Read the model definition and answer for the solid it produces. Units are mm, in the model's axes. A direction names the side the tool comes from. Give positions to 0.01 mm unless a question says otherwise; leave off trailing zeros. Write each loop counter-clockwise with the first axis right and the second up, starting at its lowest first coordinate (ties: lowest second). Pieces come first, ordered by that corner, then holes. Notation, with made-up numbers: (-25.5, 14.25) -> (23.5, 14.25) arc R21 ccw to (23.5, 28.25) -> close; hole circle Ø8 at (-33, -21.5). An arc over 180 degrees is marked (long way). Answer as CSV lines item,"result". Start each with the question number.
1. A tool of negligible diameter and unlimited length cuts with its end or side. For faces 1 (the flat face through (-2, 128, 184)), 2 (the flat face through (-150, -2, 180)), 3 (the flat face through (-153, -2, 184)), 4 (the flat face through (-3, 2, 8)), 5 (the flat face through (-171.5, 31.5, 120.2)), from which of +Z, -Z, +X, -X, +Y, -Y can it reach the whole face along a straight path? Write none if from no direction.
2. The part is cut by section D-D, the plane y = -119. Determine the outline of the cut face in (x, z).
3. Find the intervals of material crossed by line 1 (Y direction, x = 185.25, z = 145); line 2 (Y direction, x = -20, z = 146.5); line 3 (X direction, y = 103.5, z = 47), in increasing order.
4. The part is cut by section A-A, the plane z = 155.5. Determine the outline of the cut face in (x, y), and give its area (3 significant figures).
5. For a pull along Z with two mould halves and no side action, classify faces 6 (the flat face through (-3, -131, 172)), 7 (the flat face through (-2.4, -31.8, 26)), 8 (the flat face through (153, -2, 184)), 9 (the flat face through (-3, 2, 0)) as pulls with the +Z half, pulls with the -Z half, needs draft (parallel to the pull), parting line crosses it, or undercut.
6. The part is cut by section C-C, the plane x = -161. Determine the outline of the cut face in (y, z), and give its area (3 significant figures).
7. The part is cut by section B-B, the plane y = 58. Give the number of separate pieces and of enclosed holes in the cut face, and give its area (3 significant figures).
from build123d import *

# Parameters (mm, degrees)
CROQUIS1_W               = 379
CROQUIS1_H               = 316
SALIENTE_EXTRUIR1_DEPTH  = 180
VACIADO1_T               = -8
CROQUIS2_R               = 35
CORTAR_EXTRUIR4_DEPTH    = 20
CROQUIS4_R               = 45
CROQUIS4_R_2             = 40
SALIENTE_EXTRUIR4_DEPTH  = 10
CORTAR_EXTRUIR6_START    = -10
CROQUIS6_R               = 45
CORTAR_EXTRUIR6_DEPTH    = 10
CROQUIS7_R               = 24
CROQUIS7_R_2             = 21
SALIENTE_EXTRUIR9_DEPTH  = 18
CROQUIS11_W              = 363
CROQUIS11_H              = 300
CROQUIS11_W_2            = 300
CROQUIS11_H_2            = 250
SALIENTE_EXTRUIR10_DEPTH = 8
CROQUIS12_W              = 306
CROQUIS12_H              = 256
CROQUIS12_W_2            = 300
CROQUIS12_H_2            = 250
SALIENTE_EXTRUIR11_DEPTH = 8
CROQUIS20_R              = 21
CROQUIS20_R_2            = 18.5
SALIENTE_EXTRUIR19_DEPTH = 10
TALADRO_ROSCADO_M63_D    = 5


with BuildPart() as part:
    # Croquis1 → Saliente-Extruir1 (new body)
    with BuildSketch(Plane.XY):
        Rectangle(CROQUIS1_W, CROQUIS1_H)
    extrude(amount=SALIENTE_EXTRUIR1_DEPTH)

    # Vaciado1
    vaciado1_openings = [part.faces().sort_by_distance(p)[0] for p in [
        (0, 0, 180),
    ]]
    offset(amount=VACIADO1_T, openings=vaciado1_openings, kind=Kind.INTERSECTION)

    # Croquis2 → Cortar-Extruir4 (cut)
    with BuildSketch(Plane.ZY.offset(189.5)):
        with Locations((90, 58)):
            Circle(CROQUIS2_R)
    extrude(amount=-CORTAR_EXTRUIR4_DEPTH, mode=Mode.SUBTRACT)

    # Croquis4 → Saliente-Extruir4 (add)
    with BuildSketch(Plane(origin=(-181.5, 0, 0), x_dir=(0, 0, -1), z_dir=(1, 0, 0))):
        with Locations((-90, 58)):
            Circle(CROQUIS4_R)
        with Locations((-90, 58)):
            Circle(CROQUIS4_R_2, mode=Mode.SUBTRACT)
    extrude(amount=SALIENTE_EXTRUIR4_DEPTH)

    # Croquis6 → Cortar-Extruir6 (cut)
    with BuildSketch(Plane(origin=(189.5, 0, 0), x_dir=(0, 0, -1), z_dir=(1, 0, 0)).offset(CORTAR_EXTRUIR6_START)):
        with Locations((-90, 58)):
            Circle(CROQUIS6_R)
    extrude(amount=CORTAR_EXTRUIR6_DEPTH, mode=Mode.SUBTRACT)

    # Croquis7 → Saliente-Extruir9 (add)
    with BuildSketch(Plane.XY.offset(8)):
        with Locations(Location((-2.5, -53, 0), (0, 0, 180))):
            Circle(CROQUIS7_R)
        with Locations((-2.5, -53)):
            Circle(CROQUIS7_R_2, mode=Mode.SUBTRACT)
    extrude(amount=SALIENTE_EXTRUIR9_DEPTH)

    # Croquis11 → Saliente-Extruir10 (add)
    with BuildSketch(Plane.XY.offset(180)):
        Rectangle(CROQUIS11_W, CROQUIS11_H)
        Rectangle(CROQUIS11_W_2, CROQUIS11_H_2, mode=Mode.SUBTRACT)
    extrude(amount=-SALIENTE_EXTRUIR10_DEPTH)

    # Croquis12 → Saliente-Extruir11 (add)
    with BuildSketch(Plane.XY.offset(180)):
        Rectangle(CROQUIS12_W, CROQUIS12_H)
        Rectangle(CROQUIS12_W_2, CROQUIS12_H_2, mode=Mode.SUBTRACT)
    extrude(amount=SALIENTE_EXTRUIR11_DEPTH)

    # Croquis20 → Saliente-Extruir19 (add)
    with BuildSketch(Plane.XY.offset(8)):
        with Locations((-2.5, -53)):
            Circle(CROQUIS20_R)
        with Locations((-2.5, -53)):
            Circle(CROQUIS20_R_2, mode=Mode.SUBTRACT)
    extrude(amount=SALIENTE_EXTRUIR19_DEPTH)

    # Taladro roscado M63 (through all)
    with Locations(Plane(origin=(-189.5, 115.5, 35), x_dir=(0, 0, -1), z_dir=(-1, 0, 0))):
        with Locations((0, 0), (-110, 0), (-110, 115), (0, 115)):
            Hole(TALADRO_ROSCADO_M63_D / 2)


solid = part.part
Results found:
1,face 1,"+Z, +X, -X, +Y"
1,face 2,"+Z"
1,face 3,"+Z, -X, +Y, -Y"
1,face 4,"none"
1,face 5,"+X"
2,outline,"(-189.5, 0) -> (189.5, 0) -> (189.5, 180) -> (153, 180) -> (153, 188) -> (150, 188) -> (150, 172) -> (181.5, 172) -> (181.5, 8) -> (-181.5, 8) -> (-181.5, 172) -> (-150, 172) -> (-150, 188) -> (-153, 188) -> (-153, 180) -> (-189.5, 180) -> close"
3,line 1,"y = -158 to -2, 3 to 113, 118 to 158"
3,line 2,"y = -158 to -150, 150 to 158"
3,line 3,"x = -189.5 to -181.5, 181.5 to 189.5"
4,outline,"(-189.5, -158) -> (189.5, -158) -> (189.5, 158) -> (-189.5, 158) -> close; hole (-181.5, -150) -> (181.5, -150) -> (181.5, 150) -> (-181.5, 150) -> close"
4,area,"10,900 mm²"
5,face 6,"undercut"
5,face 7,"pulls with the +Z half"
5,face 8,"needs draft"
5,face 9,"pulls with the -Z half"
6,outline,"(-158, 0) -> (158, 0) -> (158, 180) -> (-158, 180) -> close; hole (-150, 8) -> (150, 8) -> (150, 172) -> (-150, 172) -> close"
6,area,"7,680 mm²"
7,separate pieces,"3"
7,enclosed holes,"0"
7,area,"5,160 mm²"
